Check sheet for the modelled part. Datum: model origin and axes. Units: mm. Face numbers are marked on the shaded views. A direction names the side the tool comes from. Round coordinates to 2 decimals unless told otherwise and drop trailing zeros. Write each loop counter-clockwise with the first axis right and the second up, starting at its lowest first coordinate (ties: lowest second). Pieces come first, ordered by that corner, then holes.
from build123d import *

# Parameters (mm, degrees)
F0_W      = 80
F0_H      = 12.5
F1_DEPTH  = 20
F2_R      = 5
F4_DEPTH  = 20
F5_R      = 5
F7_DEPTH  = 25
F9_DEPTH  = 25
F10_W     = 20
F10_H     = 0.8859829484
F11_DEPTH = 25
F13_DEPTH = 19
F14_R     = 2
F15_R     = 1.45
F16_DEPTH = 100


with BuildPart() as f1:
    # F0 (on Right) → F1 (new body)
    with BuildSketch(Plane.YZ):
        with Locations((-40, 6.25)):
            Rectangle(F0_W, F0_H)
    extrude(amount=F1_DEPTH)

    # F2
    f2_edges = [f1.edges().sort_by_distance(p)[0] for p in [
        (20, -40, 12.5),
        (20, -40, 0),
        (0, -40, 12.5),
        (0, -40, 0),
    ]]
    fillet(f2_edges, radius=F2_R)

    # F3 (on face) → F4 (join)
    with BuildSketch(Plane(origin=(0, 0, 0), x_dir=(-1, 0, 0), z_dir=(0, 1, 0))):
        Polygon((-22.5355339059, 14.0355339059), (-22.5355339059, 11.0355339059), (-22.5355339059, -1.5355339059), (-18.5355339059, -1.5355339059), (2.5355339059, -1.5355339059), (2.5355339059, 11.0355339059), (2.5355339059, 14.0355339059), align=None)
    extrude(amount=F4_DEPTH)

    # F5
    f5_edges = [f1.edges().sort_by_distance(p)[0] for p in [
        (22.535534, 10, 14.035534),
        (22.535534, 10, -1.535534),
        (-2.535534, 10, -1.535534),
        (-2.535534, 10, 14.035534),
    ]]
    fillet(f5_edges, radius=F5_R)

    # F6 (on Right) → F7 (cut)
    with BuildSketch(Plane.YZ):
        Polygon((20, 0), (0, 0), (0, -2.4886932224), (20, -2.4886932224), (23.4880913049, -2.4886932224), (23.4486758709, 14.381791465), (20, 14.381791465), (-15.4835612513, 14.381791465), (-9.843991138, 12.5039182603), (20, 2.5664176792), align=None)
    extrude(amount=F7_DEPTH, mode=Mode.SUBTRACT)

    # F8 (on face) → F9 (cut)
    with BuildSketch(Plane.YZ):
        Polygon((0, 9.2260501226), (20, 2.5664176792), (20, 13.3859829484), (0, 13.3859829484), align=None)
    extrude(amount=-F9_DEPTH, mode=Mode.SUBTRACT)

    # F10 (on face) → F11 (cut)
    with BuildSketch(Plane.YZ):
        with Locations((10, -0.4429914742)):
            Rectangle(F10_W, F10_H)
    extrude(amount=-F11_DEPTH, mode=Mode.SUBTRACT)

    # F12 (on face) → F13 (join)
    with BuildSketch(Plane.XZ.offset(80)):
        Polygon((-8, 12.5), (-8, 0), (-8, -1.5), (28, -1.5), (28, 0), (28, 14), (-8, 14), align=None)
    extrude(amount=F13_DEPTH)

    # F14
    f14_edges = [f1.edges().sort_by_distance(p)[0] for p in [
        (-8, -80, 6.25),
        (28, -89.5, 14),
        (-8, -89.5, 14),
        (10, -80, 14),
        (10, -99, 14),
        (28, -89.5, -1.5),
        (28, -99, 6.25),
        (28, -80, 6.25),
        (-8, -89.5, -1.5),
        (10, -80, -1.5),
        (10, -99, -1.5),
        (-8, -99, 6.25),
    ]]
    fillet(f14_edges, radius=F14_R)

    # F15 (on face) → F16 (cut)
    with BuildSketch(Plane.YZ.offset(28)):
        with Locations((-90.3749987483, 3.750000149)):
            Circle(F15_R)
        with Locations((2.3177627008, 3.750000149)):
            Circle(F15_R)
    extrude(amount=-F16_DEPTH, mode=Mode.SUBTRACT)


solid = f1.part
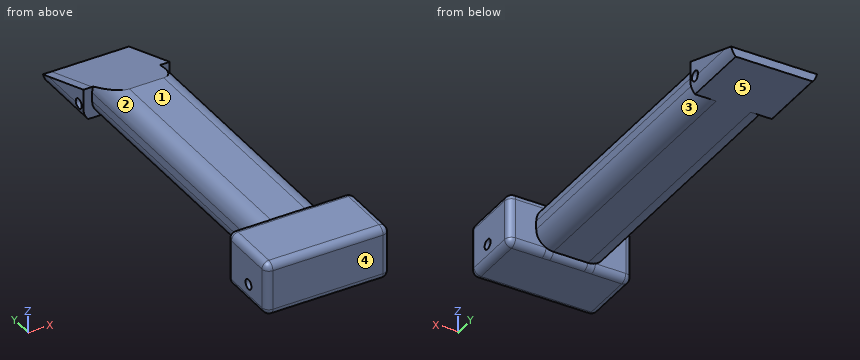
1. Scan lines: line 1 along X through (y, z) = (-12.5, 5.5); line 2 along Y through (x, z) = (25, 12); line 3 along Z through (x, y) = (6.5, -68). Record each from-to range of solid material in increasing order.
2. Sectioned sample at B-B, the plane y = -41. Enter the section's corners in (x, z).
3. Go/stop test with flat-tipped pins: pin 1 (3.5 mm diameter, centred on y = 2.32, z = 3.75, fed in from -X); pin 2 (12 mm diameter, centred on x = 24, y = -64.5, fed in from -Z); pin 3 (8 mm diameter, centred on x = -2, y = -46.5, fed in from +Z). Record where each tip stops, or that it passes through.
4. Sectioned sample at A-A, the plane z = 10.75. Enter the section's corners in (x, y), plus the area to 3 significant figures.
5. Sectioned sample at C-C, the plane y = 12.5. Enter the section's corners in (x, z), plus the area to 3 significant figures.
6. Set-up check for the marked faces 1, 2, 3, 4 and 5: record each of +Z, -Z, +X, -X, +Y, -Y from which the full face is reachable in a straight line by a thin tool's end or side.
Computed values:
1. line 1: x = 0 to 20
1. line 2: y = -99 to -80
1. line 3: z = 0 to 12.5
2. outline: (0, 5) arc R5 ccw to (5, 0) - (15, 0) arc R5 ccw to (20, 5) - (20, 7.5) arc R5 ccw to (15, 12.5) - (5, 12.5) arc R5 ccw to (0, 7.5) - close
3. pin 1: stops at x = -2.54
3. pin 2: stops at z = 1
3. pin 3: stops at z = 11.5
4. outline: (-8, -97) arc R2 ccw to (-6, -99) - (26, -99) arc R2 ccw to (28, -97) - (28, -82) arc R2 ccw to (26, -80) - (18.8, -80) - (18.8, -4.58) - (1.2, -4.58) - (1.2, -80) - (-6, -80) arc R2 ccw to (-8, -82) - close
4. area: 2,010 mm2
5. outline: (-2.54, 3.46) arc R5 ccw to (-1.14, 0) - (21.14, 0) arc R5 ccw to (22.54, 3.46) - (22.54, 5.06) - (-2.54, 5.06) - close
5. area: 124 mm2
6. face 1: +Z, +X, -X, +Y
6. face 2: +Z, -X
6. face 3: -Z, +X
6. face 4: +Z, -Z, +X, -X, -Y
6. face 5: -Z, +X, -X, +Y
